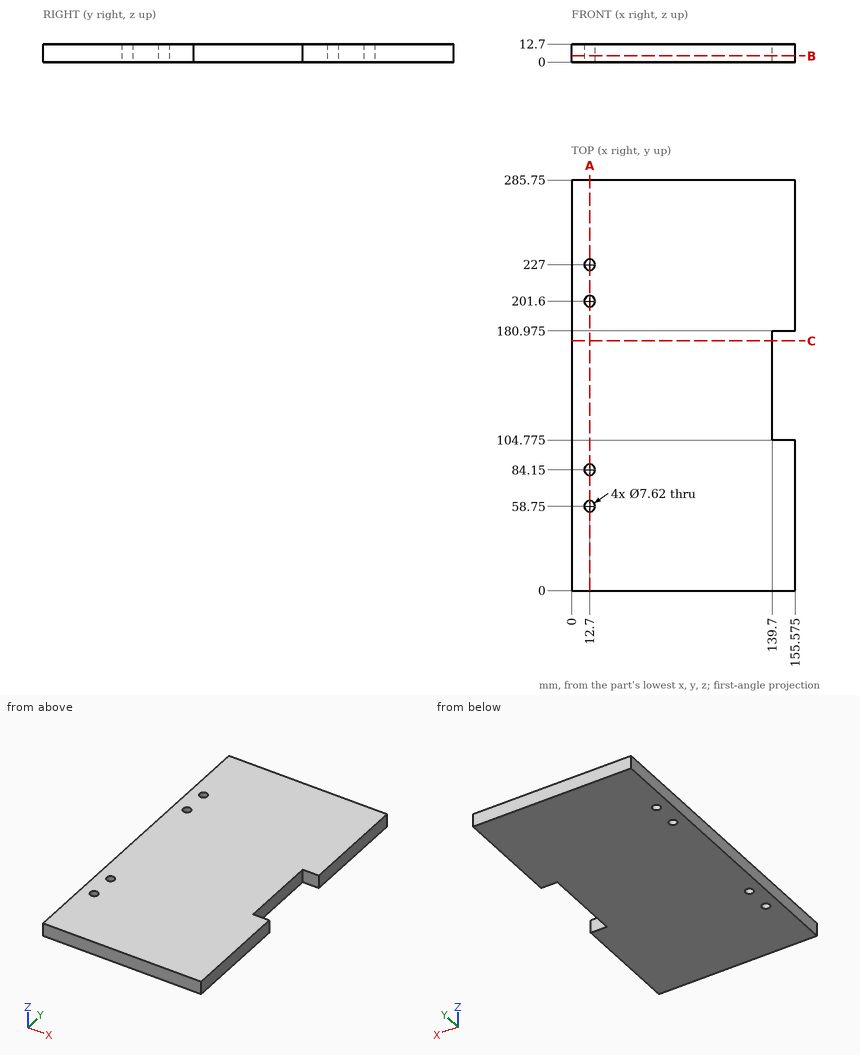
The drawing under review shows one solid part. Ordinate dimensions are in mm from its lowest x, y, z. Round coordinates to 2 decimals unless told otherwise and drop trailing zeros. Order: outer loops, then holes, each group sorted by start corner. A loop starts at its lowest first (then second) coordinate and runs counter-clockwise, first axis right, second up. Notation, with made-up numbers: (-24.75, -21.75) -> (18.25, -21.75) arc R28 ccw to (18.25, -0.75) -> close; hole circle Ø1 at (42.5, -12.5). An arc over 180 degrees is marked (long way). Use a Markdown table: item, result.
Q1. We need section B-B on z = 4.5. State how many separate pieces and enclosed holes the cut face has, then the cut area to 3 significant figures.
Values:
| item | result |
|---|---|
| separate pieces | 1 |
| enclosed holes | 4 |
| area | 43,100 mm^2 |
Q2. We need section C-C on y = 174. Write out the cut boundary in (x, z).
Values:
| item | result |
|---|---|
| outline | (0, 0) -> (139.7, 0) -> (139.7, 12.7) -> (0, 12.7) -> close |
Q3. For line 1 (Y direction, x = 12.7, z = 4.25); line 2 (Y direction, x = 140.5, z = 2.5) (3 decimals); line 3 (X direction, y = 147, z = 9.75), list the stretches that pass through material, from the lowest coordinate up.
Values:
| item | result |
|---|---|
| line 1 | y = 0 to 54.94, 62.56 to 80.34, 87.96 to 197.79, 205.41 to 223.19, 230.81 to 285.75 |
| line 2 | y = 0 to 104.775, 180.975 to 285.75 |
| line 3 | x = 0 to 139.7 |
Q4. Clearance check with a flat-ended pin moving along its axis: P1, Ø6, axis at x = 12.7, y = 227, coming from the -Z side. State where the tip first meets the part, or that it passes through.
Values:
| item | result |
|---|---|
| P1 | passes through |
Q5. We need section A-A on x = 12.7. Write out the cut boundary in (y, z), then the cut area to 3 significant figures.
Values:
| item | result |
|---|---|
| outline | (0, 0) -> (54.94, 0) -> (54.94, 12.7) -> (0, 12.7) -> close; (62.56, 0) -> (80.34, 0) -> (80.34, 12.7) -> (62.56, 12.7) -> close; (87.96, 0) -> (197.79, 0) -> (197.79, 12.7) -> (87.96, 12.7) -> close; (205.41, 0) -> (223.19, 0) -> (223.19, 12.7) -> (205.41, 12.7) -> close; (230.81, 0) -> (285.75, 0) -> (285.75, 12.7) -> (230.81, 12.7) -> close |
| area | 3,240 mm^2 |
